from build123d import *

# Parameters (mm, degrees)
BOSS_EXTRUDE1_DEPTH = 3.5
SKETCH2_R           = 1.75
CUT_EXTRUDE1_DEPTH  = 23.899960365


with BuildPart() as part:
    # Sketch1 → Boss-Extrude1 (new, symmetric)
    with BuildSketch(Plane.XY):
        with BuildLine():
            Line((-8.102202461, 9.45), (8.102202461, 9.45))
            ThreePointArc((8.102202461, 9.45), (12.447818473, 0), (8.102202461, -9.45))
            Line((8.102202461, -9.45), (-8.102202461, -9.45))
            ThreePointArc((-8.102202461, -9.45), (-12.447818473, 0), (-8.102202461, 9.45))
        make_face()
        Polygon((7.447818473, 0), (3.723909236, 6.45), (-3.723909236, 6.45), (-7.447818473, 0), (-3.723909236, -6.45), (3.723909236, -6.45), align=None, mode=Mode.SUBTRACT)
    extrude(amount=BOSS_EXTRUDE1_DEPTH, both=True)

    # Sketch2 → Cut-Extrude1 (cut, through all)
    with BuildSketch(Plane(origin=(0, 9.45, 0), x_dir=(1, 0, 0), z_dir=(0, 1, 0))):
        with Locations(Location((0, 0, 0), (0, 0, 270))):
            Circle(SKETCH2_R)
    extrude(amount=-CUT_EXTRUDE1_DEPTH, mode=Mode.SUBTRACT)


solid = part.part
Part model, mm, in its own coordinate system. A direction names the side the tool comes from. Coordinates: 2 decimals unless noted, no trailing zeros. Loops run counter-clockwise (first coordinate to the right, second up) from the corner with the lowest first, then second, coordinate; pieces in that order, holes last. Notation, with made-up numbers: (52, 26) -> (90, 26) arc R24 cw to (90, 63) -> close; hole circle Ø3 at (0, -5.75). An arc over 180 degrees is marked (long way). Use a Markdown table: item, result. Add a question column.
Item 1: Band-saw the part on A-A on x = 0. Write the cut outline in (y, z).
Item 2: Flat gauge pin, fed straight in: P1, Ø2, axis at x = -0.5, z = 0, coming from the +Y side. Where does the tip first touch, or does it go through?
Item 3: Band-saw the part on C-C on y = 5. Write the cut outline in (x, z).
Item 4: Probe probe 1 along Y at (x, z) = (-3, -2.5); probe 2 along X at (y, z) = (4.5, 1.25); probe 3 along X at (y, z) = (7.6, 0). List the from-to ranges inside material, lowest first.
Item 5: Which spindle directions (+Z, -Z, +X, -X, +Y, -Y) get a long thin tool onto all of the face, cutting with end or side? Do faces 1 (the cylindrical face through (-1.71, 7.97, -0.38)), 2 (the flat face through (5.6, 3.2, 0)). Say none if no direction does.
Item 6: Band-saw the part on B-B on z = 0. Write the cut outline in (x, y), plus the area to 3 significant figures.
Item 7: Pull direction X, two halves, no side cores. Call faces 3 (the cylindrical face through (-12.447, -0.15, 0.049)), 4 (the cylindrical face through (12.447, 0.15, 0.049)), 5 (the flat face through (-5.6, -3.2, 0)), 6 (the flat face through (6, 4, 3.5)): +X half, -X half, draft (parallel to the pull), parting line (faces both ways), or undercut.
Item 8: Band-saw the part on D-D on x = 2.75. Write the cut outline in (y, z).
Geometry says:
| question | item | result |
|---|---|---|
| 1 | outline | (-9.45, -3.5) -> (-6.45, -3.5) -> (-6.45, -1.75) -> (-9.45, -1.75) -> close; (-9.45, 1.75) -> (-6.45, 1.75) -> (-6.45, 3.5) -> (-9.45, 3.5) -> close; (6.45, -3.5) -> (9.45, -3.5) -> (9.45, -1.75) -> (6.45, -1.75) -> close; (6.45, 1.75) -> (9.45, 1.75) -> (9.45, 3.5) -> (6.45, 3.5) -> close |
| 2 | P1 | through |
| 3 | outline | (-11.4, -3.5) -> (-4.56, -3.5) -> (-4.56, 3.5) -> (-11.4, 3.5) -> close; (4.56, -3.5) -> (11.4, -3.5) -> (11.4, 3.5) -> (4.56, 3.5) -> close |
| 4 | probe 1 | -9.45 to -6.45, 6.45 to 9.45 |
| 4 | probe 2 | -11.61 to -4.85, 4.85 to 11.61 |
| 4 | probe 3 | -9.86 to -1.75, 1.75 to 9.86 |
| 5 | face 1 | +Y, -Y |
| 5 | face 2 | +Z, -Z |
| 6 | outline | (-8.1, -9.45) -> (-1.75, -9.45) -> (-1.75, -6.45) -> (-3.72, -6.45) -> (-7.45, 0) -> (-3.72, 6.45) -> (-1.75, 6.45) -> (-1.75, 9.45) -> (-8.1, 9.45) arc R12.45 ccw to start; (1.75, -9.45) -> (8.1, -9.45) arc R12.45 ccw to (8.1, 9.45) -> (1.75, 9.45) -> (1.75, 6.45) -> (3.72, 6.45) -> (7.45, 0) -> (3.72, -6.45) -> (1.75, -6.45) -> close |
| 6 | area | 255 mm² |
| 7 | face 3 | -X half |
| 7 | face 4 | +X half |
| 7 | face 5 | undercut |
| 7 | face 6 | draft |
| 8 | outline | (-9.45, -3.5) -> (-6.45, -3.5) -> (-6.45, 3.5) -> (-9.45, 3.5) -> close; (6.45, -3.5) -> (9.45, -3.5) -> (9.45, 3.5) -> (6.45, 3.5) -> close |
